Study the drawing (mm; zero at the part's minimum x, y, z) and answer. A direction names the side the tool comes from. Round coordinates to 2 decimals unless told otherwise and drop trailing zeros. Write each loop counter-clockwise with the first axis right and the second up, starting at its lowest first coordinate (ties: lowest second). Pieces come first, ordered by that corner, then holes. Notation, with made-up numbers: M 16,-26 L 71,-26 A23 ccw 71,2 Z; hole C -27.5,-4.5 d1. An arc over 180 degrees is marked long. Write each question's results on one line, items separated by ' | '.
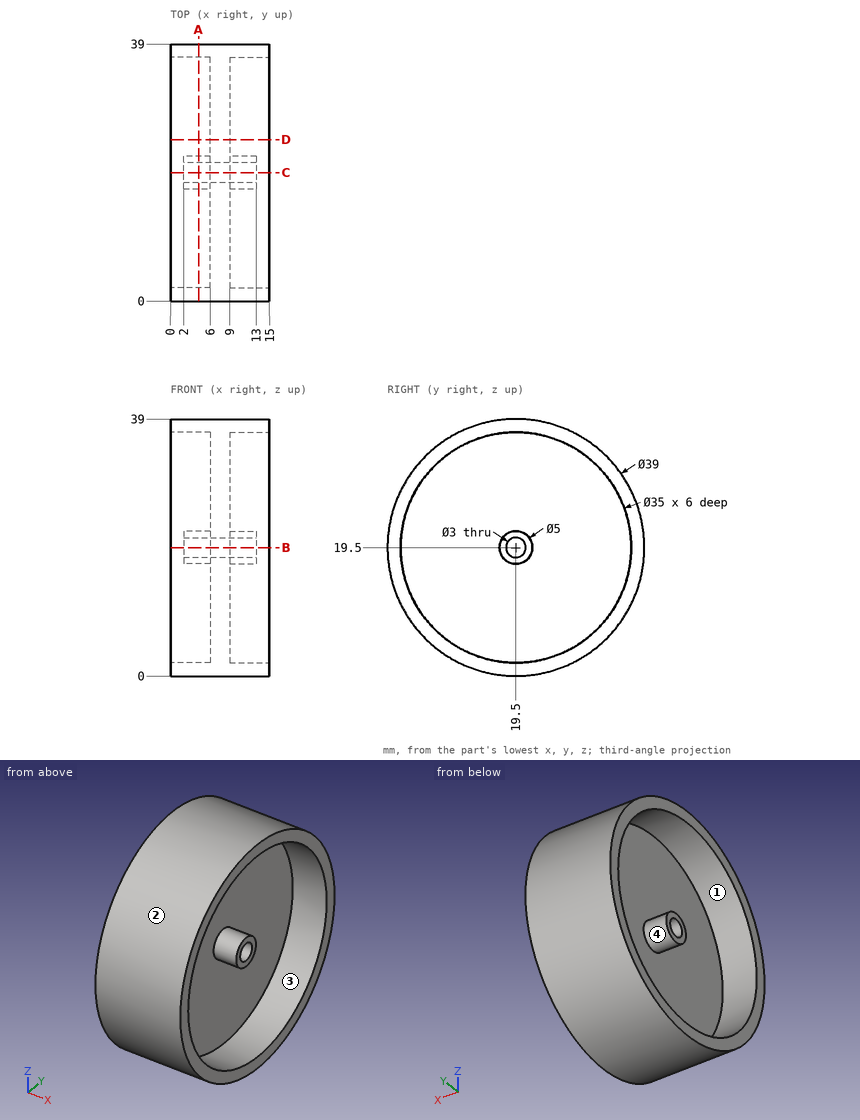
1) The mould has two halves that part along Y. Classify the marked faces 1 and 2: +Y half, -Y half, draft (parallel to the pull), parting line (faces both ways), or undercut.
Return value:
face 1: undercut | face 2: parting line
2) Section D-D (y = 24.5) is taken. Determine the outline of the cut face in (x, z).
Return value:
outline: M 0,0.65 L 15,0.65 L 15,2.73 L 9,2.73 L 9,36.27 L 15,36.27 L 15,38.35 L 0,38.35 L 0,36.27 L 6,36.27 L 6,2.73 L 0,2.73 Z
3) Section A-A (x = 4.25) is taken. Determine the outline of the cut face in (y, z).
Return value:
outline: C 19.5,19.5 d39; C 19.5,19.5 d5; hole C 19.5,19.5 d35; hole C 19.5,19.5 d3
4) Each of these flat-tipped pins is pushed along its axis until it touches: pin 1 (8 mm diameter, centred on x = 5.5, y = 20, fed in from -Z); pin 2 (1.5 mm diameter, centred on y = 10, z = 32.5, fed in from +X); pin 3 (8 mm diameter, centred on y = 25.5, z = 18, fed in from -X). Where does it stop, or does it pass through?
Return value:
pin 1: z = 0 | pin 2: x = 9 | pin 3: x = 2
5) Find the intervals of material crossed by line 1 (Z direction, x = 10.6, y = 19.5); line 2 (Z direction, x = 2.75, y = 19); line 3 (Y direction, x = 1.25, z = 19), in increasing order.
Return value:
line 1: 0 to 2, 17 to 18, 21 to 22, 37 to 39 | line 2: 0.01 to 2.01, 17.05 to 18.09, 20.91 to 21.95, 36.99 to 38.99 | line 3: 0.01 to 2.01, 36.99 to 38.99
6) Section B-B (z = 19.5) is taken. Determine the outline of the cut face in (x, y), then the cut area to 3 significant figures.
Return value:
outline: M 0,0 L 15,0 L 15,2 L 9,2 L 9,17 L 13,17 L 13,18 L 2,18 L 2,17 L 6,17 L 6,2 L 0,2 Z; M 0,37 L 6,37 L 6,22 L 2,22 L 2,21 L 13,21 L 13,22 L 9,22 L 9,37 L 15,37 L 15,39 L 0,39 Z | area: 172 mm²
7) A tool of negligible diameter and unlimited length cuts with its end or side. For the marked faces 3 and 4, from which of +Z, -Z, +X, -X, +Y, -Y can it reach the whole face along a straight path? Write none if from no direction.
Return value:
face 3: +X | face 4: -X
